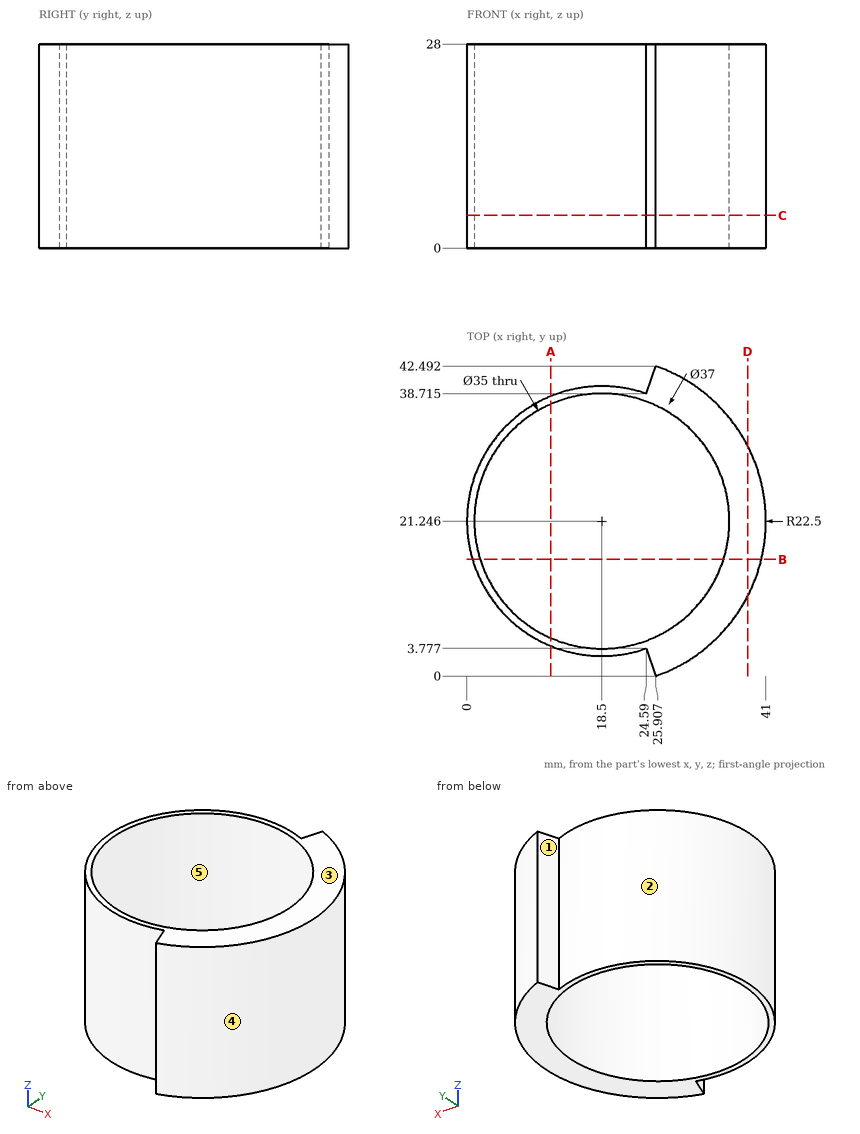
The figure shows three views and two pictorial views of one solid part (mm, origin at its lowest corner). Answer the questions. A direction names the side the tool comes from. Give positions to 0.01 mm unless a question says otherwise; leave off trailing zeros. Write each loop counter-clockwise with the first axis right and the second up, starting at its lowest first coordinate (ties: lowest second). Pieces come first, ordered by that corner, then holes. Notation, with made-up numbers: (27, -22) - (41, -22) arc R22 cw to (41, -13) - close; hole circle Ø10 at (55.25, 23). An arc over 180 degrees is marked (long way). Use one line per item in the form item = value. Start each with the question number.
1) Find section A-A on x = 11.5. Determine the outline of the cut face in (y, z) (1 decimal).
2) Find section B-B on y = 16. Determine the outline of the cut face in (x, z) (1 decimal), plus the area to 3 significant figures.
3) A tool of negligible diameter and unlimited length cuts with its end or side. For the marked faces 1 and 2, from which of +Z, -Z, +X, -X, +Y, -Y can it reach the whole face along a straight path? Write none if from no direction.
4) The mould has two halves that part along Y. Classify the marked faces 3, 4 and 5: pulls with the +Y half, pulls with the -Y half, needs draft (parallel to the pull), parting line crosses it, or undercut.
5) Find section C-C on z = 4.5. Determine the outline of the cut face in (x, y) (1 decimal).
6) Consider line 1 along X through (y, z) = (21, 3); line 2 along X through (y, z) = (24, 25.75); line 3 along Y through (x, z) = (30, 10) (1 decimal). Determine where each line is inside the solid, lowest interval first. Write a range as from..to.
7) Flat-ended cylindrical pins translate along their axes: pin 1 Ø1 at (x, z) = (15.5, 20.5) entering from +Y; pin 2 Ø1.5 at (x, y) = (4.5, 6) entering from -Z; pin 3 Ø10 at (x, z) = (10, 9.5) entering from +Y; pin 4 Ø5 at (y, z) = (37, 24.5) entering from +X. Find the tip coordinate at first contact, or state that the pin passes through.
8) Find section D-D on x = 38.5. Determine the outline of the cut face in (y, z).
Geometry results:
q1.outline = (4.1, 0) - (5.2, 0) - (5.2, 28) - (4.1, 28) - close; (37.3, 0) - (38.4, 0) - (38.4, 28) - (37.3, 28) - close
q2.outline = (0.8, 0) - (1.8, 0) - (1.8, 28) - (0.8, 28) - close; (35.2, 0) - (40.4, 0) - (40.4, 28) - (35.2, 28) - close
q2.area = 174 mm2
q3.face_1 = +Z, -Z, +Y
q3.face_2 = +Z, -Z
q4.face_3 = needs draft
q4.face_4 = parting line crosses it
q4.face_5 = undercut
q5.outline = (24.6, 3.8) - (25.9, 0) arc R22.5 ccw to (25.9, 42.5) - (24.6, 38.7) arc R18.5 ccw (long way) to start; hole circle Ø35 at (18.5, 21.2)
q6.line_1 = 0..1, 36..41
q6.line_2 = 0.21..1.22, 35.78..40.83
q6.line_3 = 1.9..8.1, 34.4..40.6
q7.pin_1 = 39.58
q7.pin_2 = through
q7.pin_3 = 39.41
q7.pin_4 = 36.68
q8.outline = (10.94, 0) - (31.55, 0) - (31.55, 28) - (10.94, 28) - close
